CAD build for the part. Positions are in the model's coordinates, mm. A direction names the side the tool comes from. Give positions to 0.01 mm unless a question says otherwise; leave off trailing zeros. Order: outer loops, then holes, each group sorted by start corner. A loop starts at its lowest first (then second) coordinate and runs counter-clockwise, first axis right, second up. Notation, with made-up numbers: (-37, 19) -> (20, 19) arc R27 ccw to (20, 56) -> close; hole circle Ø10 at (50.25, 6). An arc over 180 degrees is marked (long way). Answer as CSV lines item,"result".
```python
from build123d import *

# Parameters (mm, degrees)
ESQUISSE1_W             = 41
ESQUISSE1_H             = 10
BOSS_EXTRU_1_DEPTH      = 12
ESQUISSE2_W             = 41
ESQUISSE2_H             = 3
BOSS_EXTRU_2_DEPTH      = 10
ESQUISSE3_R             = 1.625
ENL_V_MAT_EXTRU_1_DEPTH = 10
ENL_V_MAT_EXTRU_2_DEPTH = 42


with BuildPart() as part:
    # Esquisse1 → Boss.-Extru.1 (new body)
    with BuildSketch(Plane.XY):
        with Locations((20.5, -5)):
            Rectangle(ESQUISSE1_W, ESQUISSE1_H)
    extrude(amount=BOSS_EXTRU_1_DEPTH)

    # Esquisse2 → Boss.-Extru.2 (add)
    with BuildSketch(Plane.XZ.offset(10)):
        with Locations((20.5, 1.5)):
            Rectangle(ESQUISSE2_W, ESQUISSE2_H)
    extrude(amount=BOSS_EXTRU_2_DEPTH)

    # Esquisse3 → Enlèv. mat.-Extru.1 (cut)
    with BuildSketch(Plane.XY.offset(3)):
        with Locations((5.5, -15)):
            Circle(ESQUISSE3_R)
        with Locations((35.5, -15)):
            Circle(ESQUISSE3_R)
    extrude(amount=-ENL_V_MAT_EXTRU_1_DEPTH, mode=Mode.SUBTRACT)

    # Esquisse4 → Enlèv. mat.-Extru.2 (cut, through all)
    with BuildSketch(Plane(origin=(41, 0, 0), x_dir=(0, 0, -1), z_dir=(1, 0, 0))):
        Polygon((-12, 0), (-11.4, -10), (-12, -10), align=None)
    extrude(amount=-ENL_V_MAT_EXTRU_2_DEPTH, mode=Mode.SUBTRACT)


solid = part.part
```
1) Wall check: line 1 along Y through (x, z) = (35.5, 1.25) (3 decimals); line 2 along Z through (x, y) = (20.5, -13.5); line 3 along Y through (x, z) = (16, 6.25). Give the ranges that are in metal, low to high. Write a range as [from, to].
Data:
line 1,"y = [-20, -16.625], [-13.375, 0]"
line 2,"z = [0, 3]"
line 3,"y = [-10, 0]"
2) Pin check, flat tips, straight feed: P1, Ø5, axis at x = 35.5, y = -15, coming from the +Z side; P2, Ø6, axis at x = 13.5, y = -7, coming from the +Z side; P3, Ø2.5, axis at x = 21, z = 6.5, coming from the -Y side. Stop position of each tip, or through.
Data:
P1,"stops at z = 3"
P2,"stops at z = 11.76"
P3,"stops at y = -10"
3) Band-saw the part on C-C, the plane z = 10.75. Write the cut outline in (x, y), then the cut area to 3 significant figures.
Data:
outline,"(0, -10) -> (41, -10) -> (41, 0) -> (0, 0) -> close"
area,"410 mm2"
4) Band-saw the part on B-B, the plane x = 35.5. Write the cut outline in (y, z) (3 decimals), then the cut area to 3 significant figures.
Data:
outline,"(-20, 0) -> (-16.625, 0) -> (-16.625, 3) -> (-20, 3) -> close; (-13.375, 0) -> (0, 0) -> (0, 12) -> (-10, 11.4) -> (-10, 3) -> (-13.375, 3) -> close"
area,"137 mm2"
5) Band-saw the part on D-D, the plane x = 24.5. Write the cut outline in (y, z).
Data:
outline,"(-20, 0) -> (0, 0) -> (0, 12) -> (-10, 11.4) -> (-10, 3) -> (-20, 3) -> close"
6) Pull direction X, two halves, no side cores. Call faces 1 (the flat face through (0, -8, 5)), 2 (the flat face through (20.787, -4.93, 11.704)), 3 (the flat face through (41, -8, 5)), 4 (the cylindrical face through (5.148, -16.586, 1.521)): pulls with the +X half, pulls with the -X half, needs draft (parallel to the pull), parting line crosses it, or undercut.
Data:
face 1,"pulls with the -X half"
face 2,"needs draft"
face 3,"pulls with the +X half"
face 4,"undercut"
7) Which spindle directions (+Z, -Z, +X, -X, +Y, -Y) get a long thin tool onto all of the face, cutting with end or side? Do faces 5 (the flat face through (20, -10, 7)), 6 (the flat face through (20, -20, 2)). Say none if no direction does.
Data:
face 5,"+Z, +X, -X, -Y"
face 6,"+Z, -Z, +X, -X, -Y"
8) Band-saw the part on A-A, the plane y = -15. Write the cut outline in (x, z) (3 decimals).
Data:
outline,"(0, 0) -> (3.875, 0) -> (3.875, 3) -> (0, 3) -> close; (7.125, 0) -> (33.875, 0) -> (33.875, 3) -> (7.125, 3) -> close; (37.125, 0) -> (41, 0) -> (41, 3) -> (37.125, 3) -> close"
